from build123d import *

# Parameters (mm, degrees)
BOSS_EXTRUDE1_DEPTH = 6.95
SKETCH2_R           = 3.640054945
BOSS_EXTRUDE2_DEPTH = 1
SKETCH3_R           = 2
BOSS_EXTRUDE4_DEPTH = 6.4
BOSS_EXTRUDE5_DEPTH = 2


with BuildPart() as part:
    # Sketch1 → Boss-Extrude1 (new, symmetric)
    with BuildSketch(Plane(origin=(0, 0, 0), x_dir=(1, 0, 0), z_dir=(0, 1, 0))):
        Polygon((-1, -3.5), (1, -3.5), (1, -1), (3.5, -1), (3.5, 1), (1, 1), (1, 3.5), (-1, 3.5), (-1, 1), (-3.5, 1), (-3.5, -1), (-1, -1), align=None)
    extrude(amount=BOSS_EXTRUDE1_DEPTH, both=True)

    # Sketch2 → Boss-Extrude2 (add)
    with BuildSketch(Plane(origin=(0, 6.95, 0), x_dir=(1, 0, 0), z_dir=(0, 1, 0))):
        with Locations(Location((0, 0, 0), (0, 0, 74.054604099))):
            Circle(SKETCH2_R)
    boss_extrude2 = extrude(amount=BOSS_EXTRUDE2_DEPTH)

    # Mirror1: Boss-Extrude2 across plane
    add(boss_extrude2.mirror(Plane.ZX))

    # Sketch3 → Boss-Extrude4 (add)
    with BuildSketch(Plane(origin=(0, -7.95, 0), x_dir=(1, 0, 0), z_dir=(0, 1, 0))):
        with Locations(Location((0, 0, 0), (0, 0, 270))):
            Circle(SKETCH3_R)
    extrude(amount=-BOSS_EXTRUDE4_DEPTH)

    # Sketch6 → Boss-Extrude5 (add, symmetric)
    with BuildSketch(Plane(origin=(0, 0, 0), x_dir=(0, 0, -1), z_dir=(1, 0, 0))):
        with BuildLine():
            Line((-2, 7.95), (-2.366643319, 10.14501086))
            ThreePointArc((-2.366643319, 10.14501086), (-2.45, 11.15), (-2.366643319, 12.15498914))
            Line((-2.366643319, 12.15498914), (-1.435716028, 17.728240876))
            ThreePointArc((-1.435716028, 17.728240876), (0, 18.944033198), (1.435716028, 17.728240876))
            Line((1.435716028, 17.728240876), (2.366643319, 12.15498914))
            ThreePointArc((2.366643319, 12.15498914), (2.45, 11.15), (2.366643319, 10.14501086))
            Line((2.366643319, 10.14501086), (2, 7.95))
            Line((2, 7.95), (0.884760215, 7.95))
            Line((0.884760215, 7.95), (1.281674852, 10.32623841))
            ThreePointArc((1.281674852, 10.32623841), (1.35, 11.15), (1.281674852, 11.97376159))
            Line((1.281674852, 11.97376159), (0.320476243, 17.728240876))
            ThreePointArc((0.320476243, 17.728240876), (0, 17.999626406), (-0.320476243, 17.728240876))
            Line((-0.320476243, 17.728240876), (-1.281674852, 11.97376159))
            ThreePointArc((-1.281674852, 11.97376159), (-1.35, 11.15), (-1.281674852, 10.32623841))
            Line((-1.281674852, 10.32623841), (-0.884760215, 7.95))
            Line((-0.884760215, 7.95), (-2, 7.95))
        make_face()
    extrude(amount=BOSS_EXTRUDE5_DEPTH, both=True)


solid = part.part
Design review of the part built by this model. Coordinates are the model's own, in mm. A direction names the side the tool comes from. Round coordinates to 2 decimals unless told otherwise and drop trailing zeros. Write each loop counter-clockwise with the first axis right and the second up, starting at its lowest first coordinate (ties: lowest second). Pieces come first, ordered by that corner, then holes. Notation, with made-up numbers: (-26.5, -2.5) - (9.5, -2.5) arc R21 ccw to (9.5, 5.5) - close; hole circle Ø8 at (76, 14). An arc over 180 degrees is marked (long way). Use a Markdown table: item, result. Add a question column.
1. We need section A-A (z = 0). State the section outline as (x, y) points.
2. We need section D-D (z = 3). State the section outline as (x, y) points.
3. For faces 4 (the face through (2, -6.95, 2)), 5 (the face through (-2, 6.95, -2)), 6 (the face through (0.028, 14.811, -0.808)), 7 (the face through (-2, 6.95, 2)), list the 3-axis set-ups (+Z, -Z, +X, -X, +Y, -Y) from which the entire face can be reached by the end or side of a thin tool; tool diameter is ignored.
4. Mouldability with a two-part tool opening along Z and no side actions: class faces 1 (the face through (0.028, 18.944, 0.029)), 2 (the face through (0.03, 11.16, 1.35)), 3 (the face through (2, -7.95, -1)) as +Z half, -Z half, draft (parallel to the pull), parting line (faces both ways), or undercut.
5. Clearance check with flat-ended pins moving along their axes: pin 1 (0.8 mm diameter, centred on x = 2.5, z = -1.5, fed in from -Y); pin 2 (3 mm diameter, centred on x = -2, y = -0.5, fed in from -Z); pin 3 (1.5 mm diameter, centred on x = 2, y = 6.5, fed in from -Z). State where each tip first meets the part, or that it passes through.
6. Wall thickness on probe 1 along Y at (x, z) = (1.5, 2.75); probe 2 along Z at (x, y) = (-3, 1.5); probe 3 along Z at (x, y) = (-0.25, -4): over which ranges is each line inside the solid? List them lowest first.
7. We need section B-B (y = 15). State the section outline as (x, z) points, then the cut area to 3 significant figures.
Output:
| question | item | result |
|---|---|---|
| 1 | outline | (-3.64, -7.95) - (-2, -7.95) - (-2, -14.35) - (2, -14.35) - (2, -7.95) - (3.64, -7.95) - (3.64, -6.95) - (3.5, -6.95) - (3.5, 6.95) - (3.64, 6.95) - (3.64, 7.95) - (-3.64, 7.95) - (-3.64, 6.95) - (-3.5, 6.95) - (-3.5, -6.95) - (-3.64, -6.95) - close; (-2, 18) - (2, 18) - (2, 18.94) - (-2, 18.94) - close |
| 2 | outline | (-2.06, -7.95) - (2.06, -7.95) - (2.06, -6.95) - (1, -6.95) - (1, 6.95) - (2.06, 6.95) - (2.06, 7.95) - (-2.06, 7.95) - (-2.06, 6.95) - (-1, 6.95) - (-1, -6.95) - (-2.06, -6.95) - close |
| 3 | face 4 | +Z, +X |
| 3 | face 5 | -Z, -X |
| 3 | face 6 | +X, -X |
| 3 | face 7 | +Z, -X |
| 4 | face 1 | parting line |
| 4 | face 2 | undercut |
| 4 | face 3 | draft |
| 5 | pin 1 | stops at y = -7.95 |
| 5 | pin 2 | stops at z = -3.5 |
| 5 | pin 3 | stops at z = -3.36 |
| 6 | probe 1 | y = -7.95 to -6.95, 6.95 to 7.95 |
| 6 | probe 2 | z = -1 to 1 |
| 6 | probe 3 | z = -3.5 to 3.5 |
| 7 | outline | (-2, -1.89) - (2, -1.89) - (2, -0.78) - (-2, -0.78) - close; (-2, 0.78) - (2, 0.78) - (2, 1.89) - (-2, 1.89) - close |
| 7 | area | 8.92 mm2 |
